Can you work these out from the model? Positions are in its coordinate system, mm. Face numbers are marked on the shaded views. Give positions to 0.01 mm unless a question says otherwise; leave off trailing zeros. Order: outer loops, then holes, each group sorted by start corner. A loop starts at its lowest first (then second) coordinate and runs counter-clockwise, first axis right, second up. Notation, with made-up numbers: (77, 32.5) - (130, 32.5) arc R32 ccw to (130, 60.5) - close; hole circle Ø4 at (7, 29). An arc over 180 degrees is marked (long way). Answer as a JSON object with one key per item and string values.
```python
from build123d import *

# Parameters (mm, degrees)
BOSS_EXTRUDE1_DEPTH     = 18.288
SKETCH1_W               = 18.288
SKETCH1_H               = 76.2
MORTISE_CUTS_DEPTH      = 1955.524073472
LPATTERN1_COUNT         = 5
LPATTERN1_PITCH         = 381
WINDOW_RECESS_DEPTH     = 6.35
SKETCH3_R               = 3.175
CUT_EXTRUDE4_DEPTH      = 1955.474972641
SKETCH6_R               = 3.175
CUT_EXTRUDE5_DEPTH      = 1955.474972641
LPATTERN2_COUNT         = 3
LPATTERN2_PITCH         = 134.62
LPATTERN2_COL_COUNT     = 3
LPATTERN2_COL_PITCH     = 134.62
MIRROR1_COPY_1_SKETCH_R = 3.175
MIRROR1_COPY_1_DEPTH    = 1955.474972641
MIRROR1_COPY_2_SKETCH_R = 3.175
MIRROR1_COPY_2_DEPTH    = 1955.474972641
MIRROR1_COPY_3_SKETCH_R = 3.175
MIRROR1_COPY_3_DEPTH    = 1955.474972641
MIRROR1_COPY_4_SKETCH_R = 3.175
MIRROR1_COPY_4_DEPTH    = 1955.474972641
SKETCH7_R               = 3.175
CUT_EXTRUDE6_DEPTH      = 1955.474972641
LPATTERN3_COUNT         = 2
LPATTERN3_PITCH         = 134.62
LPATTERN3_COL_COUNT     = 2
LPATTERN3_COL_PITCH     = 134.62
MIRROR2_COPY_1_SKETCH_R = 3.175
MIRROR2_COPY_1_DEPTH    = 1955.474972641
MIRROR2_COPY_2_SKETCH_R = 3.175
MIRROR2_COPY_2_DEPTH    = 1955.474972641
SKETCH8_R               = 3.175
CUT_EXTRUDE7_DEPTH      = 1955.524073472
SKETCH9_R               = 3.175
CUT_EXTRUDE8_DEPTH      = 1955.524073472
SKETCH10_R              = 3.175
CUT_EXTRUDE9_DEPTH      = 1955.524073472
SKETCH11_R              = 3.175
CUT_EXTRUDE10_DEPTH     = 1955.524073472


with BuildPart() as part:
    # Model → Boss-Extrude1 (new body)
    with BuildSketch(Plane.XY):
        with BuildLine():
            Line((797.921024484, 645.521024484), (726.078975516, 573.678975516))
            ThreePointArc((726.078975516, 573.678975516), (715.066919748, 557.198269396), (711.2, 537.757951031))
            Line((711.2, 537.757951031), (711.2, 0))
            Line((711.2, 0), (0, 0))
            Line((0, 0), (0, 1701.93973))
            ThreePointArc((0, 1701.93973), (7.439487758, 1719.900242242), (25.4, 1727.33973))
            Line((25.4, 1727.33973), (711.2, 1727.33973))
            Line((711.2, 1727.33973), (749.3, 1727.33973))
            ThreePointArc((749.3, 1727.33973), (767.260512242, 1719.900242242), (774.7, 1701.93973))
            Line((774.7, 1701.93973), (774.7, 1600.33973))
            ThreePointArc((774.7, 1600.33973), (767.260512242, 1582.379217758), (749.3, 1574.93973))
            Line((749.3, 1574.93973), (736.6, 1574.93973))
            ThreePointArc((736.6, 1574.93973), (718.639487758, 1567.500242242), (711.2, 1549.53973))
            Line((711.2, 1549.53973), (711.2, 965.2))
            ThreePointArc((711.2, 965.2), (726.078975516, 929.278975516), (762, 914.4))
            Line((762, 914.4), (863.6, 914.4))
            ThreePointArc((863.6, 914.4), (899.521024484, 899.521024484), (914.4, 863.6))
            Line((914.4, 863.6), (914.4, 711.2))
            ThreePointArc((914.4, 711.2), (899.521024484, 675.278975516), (863.6, 660.4))
            Line((863.6, 660.4), (833.842048969, 660.4))
            ThreePointArc((833.842048969, 660.4), (814.401730604, 656.533080252), (797.921024484, 645.521024484))
        make_face()
        with BuildLine():
            Line((558.8, 838.33973), (152.4, 838.33973))
            ThreePointArc((152.4, 838.33973), (116.478975516, 853.218705516), (101.6, 889.13973))
            Line((101.6, 889.13973), (101.6, 1549.53973))
            ThreePointArc((101.6, 1549.53973), (116.478975516, 1585.460754484), (152.4, 1600.33973))
            Line((152.4, 1600.33973), (558.8, 1600.33973))
            ThreePointArc((558.8, 1600.33973), (594.721024484, 1585.460754484), (609.6, 1549.53973))
            Line((609.6, 1549.53973), (609.6, 889.13973))
            ThreePointArc((609.6, 889.13973), (594.721024484, 853.218705516), (558.8, 838.33973))
        make_face(mode=Mode.SUBTRACT)
    extrude(amount=BOSS_EXTRUDE1_DEPTH)

    # Sketch1 → Mortise cuts (cut, through all)
    with BuildSketch(Plane.XY.offset(18.288)):
        with Locations((673.1, 88.9)):
            Rectangle(SKETCH1_W, SKETCH1_H)
        with Locations((38.1, 88.9)):
            Rectangle(SKETCH1_W, SKETCH1_H)
    mortise_cuts = extrude(amount=-MORTISE_CUTS_DEPTH, mode=Mode.SUBTRACT)

    # LPattern1: Mortise cuts ×5
    with Locations(*[(0, i * LPATTERN1_PITCH, 0) for i in range(1, LPATTERN1_COUNT)]):
        add(mortise_cuts, mode=Mode.SUBTRACT)

    # Sketch2 → Window Recess (cut)
    with BuildSketch(Plane.XY.offset(18.288)):
        with BuildLine():
            Line((635, 889.13973), (635, 1549.53973))
            ThreePointArc((635, 1549.53973), (612.681536726, 1603.421266726), (558.8, 1625.73973))
            Line((558.8, 1625.73973), (152.4, 1625.73973))
            ThreePointArc((152.4, 1625.73973), (98.518463274, 1603.421266726), (76.2, 1549.53973))
            Line((76.2, 1549.53973), (76.2, 889.13973))
            ThreePointArc((76.2, 889.13973), (98.518463274, 835.258193274), (152.4, 812.93973))
            Line((152.4, 812.93973), (558.8, 812.93973))
            ThreePointArc((558.8, 812.93973), (612.681536726, 835.258193274), (635, 889.13973))
        make_face()
    extrude(amount=-WINDOW_RECESS_DEPTH, mode=Mode.SUBTRACT)

    # Sketch3 → Cut-Extrude4 (cut, through all)
    with BuildSketch(Plane.XY.offset(11.938)):
        with Locations((105.582684355, 1592.867273145)):
            Circle(SKETCH3_R)
        with Locations((605.617315645, 1592.867273145)):
            Circle(SKETCH3_R)
        with Locations((605.617315645, 845.812186855)):
            Circle(SKETCH3_R)
        with Locations((105.582684355, 845.812186855)):
            Circle(SKETCH3_R)
    extrude(amount=-CUT_EXTRUDE4_DEPTH, mode=Mode.SUBTRACT)

    # Sketch6 → Cut-Extrude5 (cut, through all)
    with BuildSketch(Plane.XY.offset(11.938)):
        with Locations((88.9, 1219.33973)):
            Circle(SKETCH6_R)
    cut_extrude5 = extrude(amount=-CUT_EXTRUDE5_DEPTH, mode=Mode.SUBTRACT)

    # LPattern2: Cut-Extrude5 ×3
    with Locations(*[(0, -i * LPATTERN2_PITCH, 0) for i in range(1, LPATTERN2_COUNT)]):
        add(cut_extrude5, mode=Mode.SUBTRACT)

    # LPattern2 col: Cut-Extrude5 ×3
    with Locations(*[(0, i * LPATTERN2_COL_PITCH, 0) for i in range(1, LPATTERN2_COL_COUNT)]):
        add(cut_extrude5, mode=Mode.SUBTRACT)

    # Mirror1: Cut-Extrude5 across plane
    add(cut_extrude5.mirror(Plane.ZY.offset(-355.6)), mode=Mode.SUBTRACT)

    # Mirror1 copy 1 sketch → Mirror1 copy 1 (cut, through all)
    with BuildSketch(Plane(origin=(711.2, -134.62, 11.938), x_dir=(-1, 0, 0), z_dir=(0, 0, 1))):
        with Locations((88.9, -1219.33973)):
            Circle(MIRROR1_COPY_1_SKETCH_R)
    extrude(amount=-MIRROR1_COPY_1_DEPTH, mode=Mode.SUBTRACT)

    # Mirror1 copy 2 sketch → Mirror1 copy 2 (cut, through all)
    with BuildSketch(Plane(origin=(711.2, -269.24, 11.938), x_dir=(-1, 0, 0), z_dir=(0, 0, 1))):
        with Locations((88.9, -1219.33973)):
            Circle(MIRROR1_COPY_2_SKETCH_R)
    extrude(amount=-MIRROR1_COPY_2_DEPTH, mode=Mode.SUBTRACT)

    # Mirror1 copy 3 sketch → Mirror1 copy 3 (cut, through all)
    with BuildSketch(Plane(origin=(711.2, 134.62, 11.938), x_dir=(-1, 0, 0), z_dir=(0, 0, 1))):
        with Locations((88.9, -1219.33973)):
            Circle(MIRROR1_COPY_3_SKETCH_R)
    extrude(amount=-MIRROR1_COPY_3_DEPTH, mode=Mode.SUBTRACT)

    # Mirror1 copy 4 sketch → Mirror1 copy 4 (cut, through all)
    with BuildSketch(Plane(origin=(711.2, 269.24, 11.938), x_dir=(-1, 0, 0), z_dir=(0, 0, 1))):
        with Locations((88.9, -1219.33973)):
            Circle(MIRROR1_COPY_4_SKETCH_R)
    extrude(amount=-MIRROR1_COPY_4_DEPTH, mode=Mode.SUBTRACT)

    # Sketch7 → Cut-Extrude6 (cut, through all)
    with BuildSketch(Plane.XY.offset(11.938)):
        with Locations((355.6, 1613.03973)):
            Circle(SKETCH7_R)
    cut_extrude6 = extrude(amount=-CUT_EXTRUDE6_DEPTH, mode=Mode.SUBTRACT)

    # LPattern3: Cut-Extrude6 ×2
    with Locations(*[(i * LPATTERN3_PITCH, 0, 0) for i in range(1, LPATTERN3_COUNT)]):
        add(cut_extrude6, mode=Mode.SUBTRACT)

    # LPattern3 col: Cut-Extrude6 ×2
    with Locations(*[(-i * LPATTERN3_COL_PITCH, 0, 0) for i in range(1, LPATTERN3_COL_COUNT)]):
        add(cut_extrude6, mode=Mode.SUBTRACT)

    # Mirror2: Cut-Extrude6 across plane
    add(cut_extrude6.mirror(Plane(origin=(0, 1219.33973, 0), x_dir=(0, 0, 1), z_dir=(0, -1, 0))), mode=Mode.SUBTRACT)

    # Mirror2 copy 1 sketch → Mirror2 copy 1 (cut, through all)
    with BuildSketch(Plane(origin=(134.62, 2438.67946, 11.938), x_dir=(1, 0, 0), z_dir=(0, 0, 1))):
        with Locations((355.6, -1613.03973)):
            Circle(MIRROR2_COPY_1_SKETCH_R)
    extrude(amount=-MIRROR2_COPY_1_DEPTH, mode=Mode.SUBTRACT)

    # Mirror2 copy 2 sketch → Mirror2 copy 2 (cut, through all)
    with BuildSketch(Plane(origin=(-134.62, 2438.67946, 11.938), x_dir=(1, 0, 0), z_dir=(0, 0, 1))):
        with Locations((355.6, -1613.03973)):
            Circle(MIRROR2_COPY_2_SKETCH_R)
    extrude(amount=-MIRROR2_COPY_2_DEPTH, mode=Mode.SUBTRACT)

    # Sketch8 → Cut-Extrude7 (cut, through all)
    with BuildSketch(Plane.XY.offset(18.288)):
        with Locations((558.8, 774.7)):
            Circle(SKETCH8_R)
        with Locations((457.2, 774.7)):
            Circle(SKETCH8_R)
        with Locations((355.6, 774.7)):
            Circle(SKETCH8_R)
        with Locations((254, 774.7)):
            Circle(SKETCH8_R)
        with Locations((152.4, 774.7)):
            Circle(SKETCH8_R)
        with Locations((558.8, 19.05)):
            Circle(SKETCH8_R)
        with Locations((457.2, 19.05)):
            Circle(SKETCH8_R)
        with Locations((355.6, 19.05)):
            Circle(SKETCH8_R)
        with Locations((254, 19.05)):
            Circle(SKETCH8_R)
        with Locations((152.4, 19.05)):
            Circle(SKETCH8_R)
    extrude(amount=-CUT_EXTRUDE7_DEPTH, mode=Mode.SUBTRACT)

    # Sketch9 → Cut-Extrude8 (cut, through all)
    with BuildSketch(Plane(origin=(0, 0, 0), x_dir=(-1, 0, 0), z_dir=(0, 0, -1))):
        with Locations((-774.7, 858.012)):
            Circle(SKETCH9_R)
        with Locations((-854.456, 858.012)):
            Circle(SKETCH9_R)
        with Locations((-694.944, 858.012)):
            Circle(SKETCH9_R)
        with Locations((-694.944, 787.4)):
            Circle(SKETCH9_R)
        with Locations((-694.944, 716.788)):
            Circle(SKETCH9_R)
        with Locations((-774.7, 716.788)):
            Circle(SKETCH9_R)
        with Locations((-854.456, 716.788)):
            Circle(SKETCH9_R)
        with Locations((-854.456, 787.4)):
            Circle(SKETCH9_R)
    extrude(amount=-CUT_EXTRUDE8_DEPTH, mode=Mode.SUBTRACT)

    # Sketch10 → Cut-Extrude9 (cut, through all)
    with BuildSketch(Plane(origin=(0, 0, 0), x_dir=(-1, 0, 0), z_dir=(0, 0, -1))):
        with Locations((-555.244, 1657.48973)):
            Circle(SKETCH10_R)
        with Locations((-453.644, 1657.48973)):
            Circle(SKETCH10_R)
        with Locations((-352.044, 1657.48973)):
            Circle(SKETCH10_R)
        with Locations((-250.444, 1657.48973)):
            Circle(SKETCH10_R)
        with Locations((-148.844, 1657.48973)):
            Circle(SKETCH10_R)
    extrude(amount=-CUT_EXTRUDE9_DEPTH, mode=Mode.SUBTRACT)

    # Sketch11 → Cut-Extrude10 (cut, through all)
    with BuildSketch(Plane(origin=(0, 0, 0), x_dir=(-1, 0, 0), z_dir=(0, 0, -1))):
        with Locations((-711.2, 1683.548964167)):
            Circle(SKETCH11_R)
        with Locations((-711.2, 1618.524964167)):
            Circle(SKETCH11_R)
    extrude(amount=-CUT_EXTRUDE10_DEPTH, mode=Mode.SUBTRACT)


solid = part.part
```
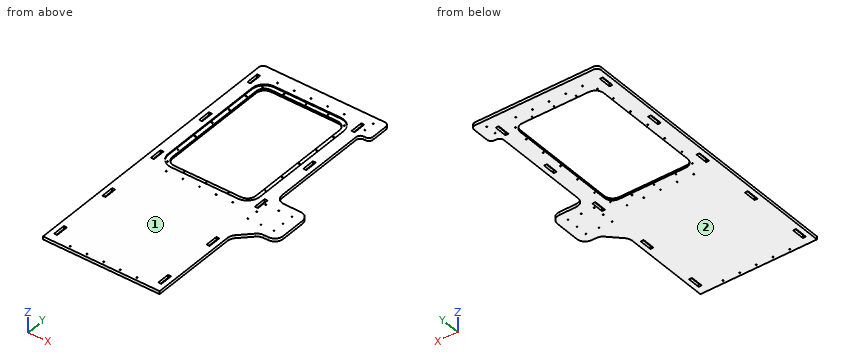
Q1. I'm going to push flat-ended pins straight in: pin 1 Ø4 at (x, y) = (605.62, 1592.87) entering from +Z; pin 2 Ø1.5 at (x, z) = (778, 11) entering from +Y; pin 3 Ø5 at (y, z) = (1294, 12) entering from +X. Where does each tip first touch, or does it pass through?
Recorded:
{"pin 1": "passes through", "pin 2": "stops at y = 914.4", "pin 3": "stops at x = 711.2"}
Q2. If we section it at A-A, the plane x = 303: Please give me the cut outline in (y, z), then the cut area to 3 significant figures.
Recorded:
{"outline": "(0, 0) - (838.34, 0) - (838.34, 11.94) - (812.94, 11.94) - (812.94, 18.29) - (0, 18.29) - close; (1600.34, 0) - (1727.34, 0) - (1727.34, 18.29) - (1625.74, 18.29) - (1625.74, 11.94) - (1600.34, 11.94) - close", "area": "17,300 mm^2"}
Q3. If we section it at C-C, the plane z = 15.5: Count the separate pieces of the cut face and the enclosed holes in it, then the cut area to 3 significant figures.
Recorded:
{"separate pieces": "1", "enclosed holes": "36", "area": "830,000 mm^2"}
Q4. We'd pull the mould along Z, two halves only. Please class the marked faces 1 and 2: released by +Z, released by -Z, zero draft, split by the parting line, or undercut.
Recorded:
{"face 1": "released by +Z", "face 2": "released by -Z"}
Q5. I need wall thicknesses on L1, parallel to X at y = 487, z = 4.25; L2, parallel to Y at x = 88.9, z = 8.5; L3, parallel to Y at x = 457.2, z = 9 (3 decimals). Which ranges of each line are inside material? Lowest first, please.
Recorded:
{"L1": "x = 0 to 28.96, 47.24 to 663.96, 682.24 to 711.2", "L2": "y = 0 to 946.92, 953.27 to 1081.54, 1087.89 to 1216.16, 1222.51 to 1350.78, 1357.13 to 1485.4, 1491.75 to 1727.34", "L3": "y = 0 to 15.875, 22.225 to 771.525, 777.875 to 838.34, 1600.34 to 1727.34"}
Q6. If we section it at B-B, the plane y = 1149: Please give me the cut outline in (x, z).
Recorded:
{"outline": "(0, 0) - (101.6, 0) - (101.6, 11.94) - (76.2, 11.94) - (76.2, 18.29) - (0, 18.29) - close; (609.6, 0) - (711.2, 0) - (711.2, 18.29) - (635, 18.29) - (635, 11.94) - (609.6, 11.94) - close"}
